Can you work these out from the model? Positions are in its coordinate system, mm. A direction names the side the tool comes from. Give positions to 0.01 mm unless a question says otherwise; leave off trailing zeros. Write each loop counter-clockwise with the first axis right and the second up, starting at its lowest first coordinate (ties: lowest second). Pieces come first, ordered by that corner, then holes.
```python
from build123d import *

# Parameters (mm, degrees)
F0_W      = 150.558009
F0_H      = 148.838363
F1_DEPTH  = 13.208
F2_W      = 126.540639
F2_H      = 125.973191
F3_DEPTH  = 14.478
F4_R      = 8.114688
F4_R_2    = 8.169072
F4_R_3    = 8.227981
F4_R_4    = 7.949321
F5_DEPTH  = 70.866
F6_W      = 133.349993
F6_H      = 132.782564
F7_DEPTH  = 17.526
F8_W      = 151.792019
F8_H      = 150.94085
F9_DEPTH  = 7.874
F10_W     = 12.939997
F10_H     = 12.656048
F10_W_2   = 13.507895
F10_H_2   = 12.779001
F10_W_3   = 13.062272
F10_W_4   = 13.346217
F10_H_3   = 11.8042
F11_DEPTH = 12.7
F12_R     = 6.673109
F13_DEPTH = 127
F14_R     = 6.64679
F15_DEPTH = 125.476
F16_R     = 5.888986
F17_DEPTH = 124.968


with BuildPart() as f1:
    # F0 (on Top) → F1 (new body)
    with BuildSketch(Plane.XY):
        with Locations((-0.219747, 0.380617)):
            Rectangle(F0_W, F0_H)
    extrude(amount=-F1_DEPTH)

    # F2 (on face) → F3 (join)
    with BuildSketch(Plane.XY):
        with Locations((-0.567448, 0.567446)):
            Rectangle(F2_W, F2_H)
    extrude(amount=F3_DEPTH)

    # F4 (on face) → F5 (join)
    with BuildSketch(Plane.XY.offset(14.478)):
        with Locations((-53.907447, 54.758616)):
            Circle(F4_R)
        with Locations((-54.474894, -53.340003)):
            Circle(F4_R_2)
        with Locations((53.623725, -53.056277)):
            Circle(F4_R_3)
        with Locations((53.907447, 54.758616)):
            Circle(F4_R_4)
    extrude(amount=F5_DEPTH)

    # F6 (on face) → F7 (join)
    with BuildSketch(Plane.XY.offset(85.344)):
        with Locations((-0.567448, 0.851169)):
            Rectangle(F6_W, F6_H)
    extrude(amount=F7_DEPTH)

    # F8 (on face) → F9 (join)
    with BuildSketch(Plane.XY.offset(102.87)):
        with Locations((-0.425584, 0.851169)):
            Rectangle(F8_W, F8_H)
    extrude(amount=F9_DEPTH)

    # F10 (on face) → F11 (join)
    with BuildSketch(Plane.XY.offset(110.744)):
        with Locations((-69.851596, 69.99357)):
            Rectangle(F10_W, F10_H)
        with Locations((-69.567646, -68.229755)):
            Rectangle(F10_W_2, F10_H_2)
        with Locations((68.939289, -68.229755)):
            Rectangle(F10_W_3, F10_H_2)
        with Locations((68.797316, 70.419494)):
            Rectangle(F10_W_4, F10_H_3)
    extrude(amount=F11_DEPTH)

    # F12 (on face) → F13 (join)
    with BuildSketch(Plane.XZ.offset(-64.517394)):
        with Locations((68.797316, 117.094)):
            Circle(F12_R)
    extrude(amount=F13_DEPTH)

    # F14 (on face) → F15 (join)
    with BuildSketch(Plane.XZ.offset(-63.665546)):
        with Locations((-69.674805, 117.219515)):
            Circle(F14_R)
    extrude(amount=F15_DEPTH)

    # F16 (on face) → F17 (join)
    with BuildSketch(Plane.YZ.offset(-62.813699)):
        with Locations((-68.470404, 117.315501)):
            Circle(F16_R)
    extrude(amount=F17_DEPTH)


solid = f1.part
```
1) Suppose I cut it at D-D on y = -49.5. Write out the boundary of the cut face in (x, z).
Values follow:
outline: (-76.32, 102.87) - (-67.24, 102.87) - (-67.24, 85.34) - (-61.69, 85.34) - (-61.69, 14.48) - (-63.84, 14.48) - (-63.84, 0) - (-75.5, 0) - (-75.5, -13.21) - (75.06, -13.21) - (75.06, 0) - (62.7, 0) - (62.7, 14.48) - (61.04, 14.48) - (61.04, 85.34) - (66.11, 85.34) - (66.11, 102.87) - (75.47, 102.87) - (75.47, 110.74) - (70.85, 110.74) arc R6.67 ccw (long way) to (66.75, 110.74) - (-68.18, 110.74) arc R6.65 ccw (long way) to (-71.17, 110.74) - (-76.32, 110.74) - close; hole (-47.26, 14.48) - (46.2, 14.48) - (46.2, 85.34) - (-47.26, 85.34) - close
2) For pin 1 Ø16 at (y, z) = (0.5, 7.5) entering from -X; pin 2 Ø3 at (y, z) = (17.5, 98.5) entering from +X; pin 3 Ø6 at (x, y) = (-19, 32.5) entering from +Z, each with a flat end and sliding along its axis, tell me the tip position at first contact or that it passes through.
Values follow:
pin 1: stops at x = -75.5
pin 2: stops at x = 66.11
pin 3: stops at z = 110.74
3) Suppose I cut it at B-B on x = 52.5. Write out the boundary of the cut face in (y, z), plus the area to 3 significant figures.
Values follow:
outline: (-74.62, 102.87) - (-65.54, 102.87) - (-65.54, 85.34) - (-61.21, 85.34) - (-61.21, 14.48) - (-62.42, 14.48) - (-62.42, 0) - (-74.04, 0) - (-74.04, -13.21) - (74.8, -13.21) - (74.8, 0) - (63.55, 0) - (63.55, 14.48) - (62.58, 14.48) - (62.58, 85.34) - (67.24, 85.34) - (67.24, 102.87) - (76.32, 102.87) - (76.32, 110.74) - (-74.62, 110.74) - close; circle Ø11.78 at (-68.47, 117.32); hole (-44.91, 14.48) - (46.93, 14.48) - (46.93, 85.34) - (-44.91, 85.34) - close
area: 9,680 mm2
4) For faces 1 (the face through (-1.2, -73.14, 113.73)), 2 (the face through (74, 64.517, 112)), 3 (the face through (-75, 63.666, 122)), which set-ups out of +Z, -Z, +X, -X, +Y, -Y let a thin tool reach every point of the face, with its end or its side?
Values follow:
face 1: none
face 2: +X
face 3: +Z, -X
5) Suppose I cut it at A-A on y = 11. Write out the boundary of the cut face in (x, z), plus the area to 3 significant figures.
Values follow:
outline: (-76.32, 102.87) - (-67.24, 102.87) - (-67.24, 85.34) - (66.11, 85.34) - (66.11, 102.87) - (75.47, 102.87) - (75.47, 110.74) - (70.85, 110.74) arc R6.67 ccw (long way) to (66.75, 110.74) - (-68.18, 110.74) arc R6.65 ccw (long way) to (-71.17, 110.74) - (-76.32, 110.74) - close; (-75.5, -13.21) - (75.06, -13.21) - (75.06, 0) - (62.7, 0) - (62.7, 14.48) - (-63.84, 14.48) - (-63.84, 0) - (-75.5, 0) - close
area: 7,630 mm2
6) Suppose I cut it at C-C on x = -41. Write out the boundary of the cut face in (y, z), plus the area to 3 significant figures.
Values follow:
outline: (-74.62, 102.87) - (-65.54, 102.87) - (-65.54, 85.34) - (67.24, 85.34) - (67.24, 102.87) - (76.32, 102.87) - (76.32, 110.74) - (-74.62, 110.74) - close; circle Ø11.78 at (-68.47, 117.32); (-74.04, -13.21) - (74.8, -13.21) - (74.8, 0) - (63.55, 0) - (63.55, 14.48) - (-62.42, 14.48) - (-62.42, 0) - (-74.04, 0) - close
area: 7,410 mm2
7) If we mould it in two halves opening along X, with no side actions, what happens to faces 4 (the face through (66.108, 0, 94)), 5 (the face through (-1, -74.039, -7)), 6 (the face through (-64, 63.666, 122)), 7 (the face through (58.05, -46.12, 49.41))? For each: +X half, -X half, draft (parallel to the pull), parting line (faces both ways), or undercut.
Values follow:
face 4: +X half
face 5: draft
face 6: undercut
face 7: undercut
8) Please list where these lines run through material, in increasing order: L1, parallel to Z at x = -47, y = 44.5; L2, parallel to Z at x = -65, y = 44.5; L3, parallel to X at y = -39, z = 117.
Values follow:
L1: z = -13.21 to 14.48, 85.34 to 110.74
L2: z = -13.21 to 0, 85.34 to 110.74, 112.49 to 121.94
L3: x = -76.32 to -63.03, 62.12 to 75.47
